Verification items for the finished model (mm, model axes). Round coordinates to 2 decimals unless told otherwise and drop trailing zeros. Write each loop counter-clockwise with the first axis right and the second up, starting at its lowest first coordinate (ties: lowest second). Pieces come first, ordered by that corner, then holes. Notation, with made-up numbers: M -40,15 L 18,15 A36 ccw 18,51 Z; hole C 59,50.5 d3. An arc over 180 degrees is marked long. One line per item, written item: value. Start each with the question number.
Item 1: Gauge pin test, flat ends, axial feed: pin 1 (12 mm diameter, centred on x = -11, y = -17, fed in from +Z); pin 2 (1 mm diameter, centred on x = -15, y = -13, fed in from -Z); pin 3 (1.5 mm diameter, centred on x = -27.5, z = 1.5, fed in from +Y). Record the tip position at first contact, or that the pin passes through.
Item 2: Section check B-B, the plane y = 0. Record the cut outline in (x, z).
Item 3: Section check D-D, the plane y = -17. Record the cut outline in (x, z).
Item 4: Section check A-A, the plane z = 1.5. Record the cut outline in (x, y).
Item 5: Section check C-C, the plane x = 0. Record the cut outline in (y, z).
Item 6: Thickness scan on probe 1 along Y at (x, z) = (0, 0.6); probe 2 along X at (y, z) = (5, 0.7); probe 3 along X at (y, z) = (8, 1.2). Record the ranges inside material, lowest first. Write a range as from..to.
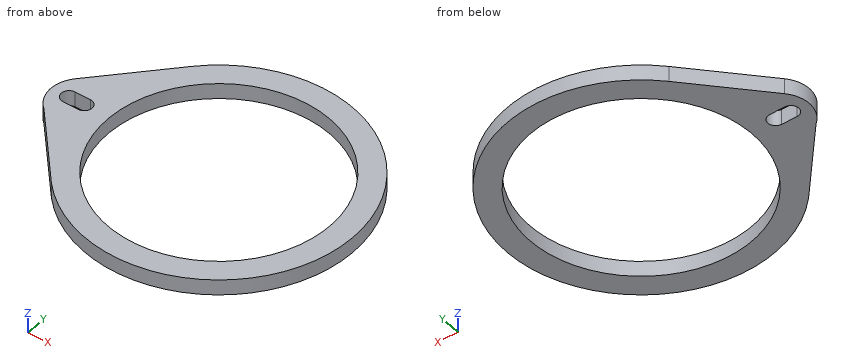
from build123d import *

# Parameters (mm, degrees)
EXTRUDE_1_DEPTH     = 3
SKETCH_2_R          = 21.5
CUT_EXTRUDE_1_DEPTH = 10


with BuildPart() as part:
    # 스케치1 → 보스-돌출1 (new body)
    with BuildSketch(Plane.XY):
        with BuildLine():
            Line((-19.259259259, 17.466566142), (-31.444444444, 4.030746033))
            ThreePointArc((-31.444444444, 4.030746033), (-32.981389073, -0.472212618), (-30.756898072, -4.678217276))
            Line((-30.756898072, -4.678217276), (-18.61420291, -18.152450249))
            ThreePointArc((-18.61420291, -18.152450249), (25.995737465, 0.470779859), (-19.259259259, 17.466566142))
        make_face()
    extrude(amount=EXTRUDE_1_DEPTH)

    # 스케치2 → 컷-돌출1 (cut)
    with BuildSketch(Plane(origin=(0, 0, 0), x_dir=(-1, 0, 0), z_dir=(0, 0, -1))):
        Circle(SKETCH_2_R)
        with BuildLine():
            Line((26.5, 1.5), (29.5, 1.5))
            ThreePointArc((29.5, 1.5), (31, 0), (29.5, -1.5))
            Line((29.5, -1.5), (26.5, -1.5))
            ThreePointArc((26.5, -1.5), (25, 0), (26.5, 1.5))
        make_face()
    extrude(amount=-CUT_EXTRUDE_1_DEPTH, mode=Mode.SUBTRACT)


solid = part.part
Response values:
1. pin 1: stops at z = 3
1. pin 2: passes through
1. pin 3: stops at y = 9.21
2. outline: M -33,0 L -31,0 L -31,3 L -33,3 Z; M -25,0 L -21.5,0 L -21.5,3 L -25,3 Z; M 21.5,0 L 26,0 L 26,3 L 21.5,3 Z
3. outline: M -19.65,0 L -13.16,0 L -13.16,3 L -19.65,3 Z; M 13.16,0 L 19.67,0 L 19.67,3 L 13.16,3 Z
4. outline: M -31.44,4.03 A6 ccw -30.76,-4.68 L -18.61,-18.15 A26 ccw long -19.26,17.47 Z; hole M -29.5,-1.5 L -26.5,-1.5 A1.5 ccw -26.5,1.5 L -29.5,1.5 A1.5 ccw Z; hole C 0,0 d43
5. outline: M -26,0 L -21.5,0 L -21.5,3 L -26,3 Z; M 21.5,0 L 26,0 L 26,3 L 21.5,3 Z
6. probe 1: y = -26..-21.5, 21.5..26
6. probe 2: x = -30.57..-20.91, 20.91..25.51
6. probe 3: x = -27.84..-19.96, 19.96..24.74
